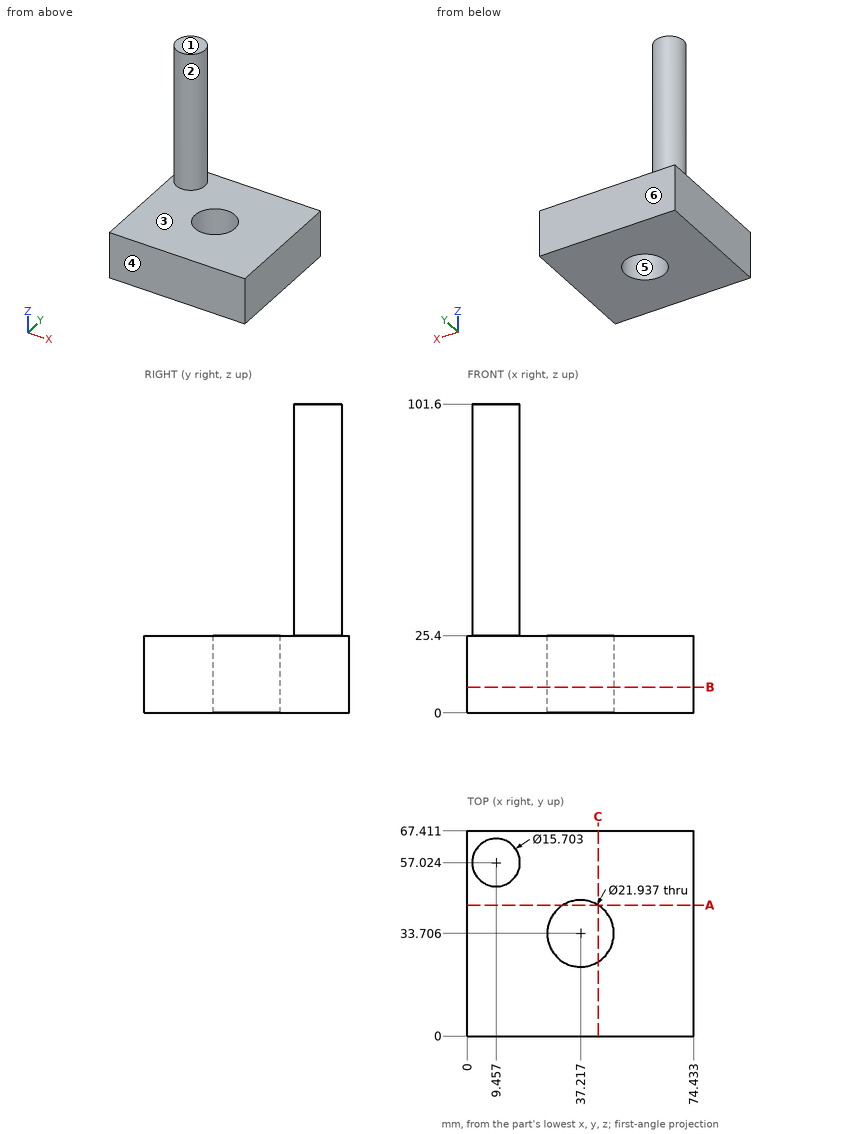
Here's the drawing with two shaded views (mm, measured from the low corner). I have some questions. A direction names the side the tool comes from. Coordinates: 2 decimals unless noted, no trailing zeros. Order: outer loops, then holes, each group sorted by start corner. A loop starts at its lowest first (then second) coordinate and runs counter-clockwise, first axis right, second up.
Item 1: If we mould it in two halves opening along Y, with no side actions, what happens to the marked faces 3, 4, 5 and 6? For each: +Y half, -Y half, draft (parallel to the pull), parting line (faces both ways), or undercut.
Result sheet:
face 3: draft
face 4: -Y half
face 5: undercut
face 6: +Y half
Item 2: If we section it at B-B on z = 8.5: List the corners of the cut face in (x, y) for me (1 decimal).
Result sheet:
outline: (0, 0) - (74.4, 0) - (74.4, 67.4) - (0, 67.4) - close; hole circle Ø21.9 at (37.2, 33.7)
Item 3: If we section it at C-C on x = 43: List the corners of the cut face in (y, z) for me (1 decimal), plus the area to 3 significant figures.
Result sheet:
outline: (0, 0) - (24.4, 0) - (24.4, 25.4) - (0, 25.4) - close; (43, 0) - (67.4, 0) - (67.4, 25.4) - (43, 25.4) - close
area: 1,240 mm2
Item 4: If we section it at A-A on y = 43: List the corners of the cut face in (x, z) for me, plus the area to 3 significant figures.
Result sheet:
outline: (0, 0) - (31.39, 0) - (31.39, 25.4) - (0, 25.4) - close; (43.04, 0) - (74.43, 0) - (74.43, 25.4) - (43.04, 25.4) - close
area: 1,590 mm2
Item 5: For the marked faces 1 and 2, which set-ups out of +Z, -Z, +X, -X, +Y, -Y let a thin tool reach every point of the face, with its end or its side?
Result sheet:
face 1: +Z, +X, -X, +Y, -Y
face 2: +Z
Item 6: I need wall thicknesses on line 1 (Z direction, x = 71, y = 18); line 2 (Y direction, x = 12.5, z = 66) (1 decimal); line 3 (X direction, y = 55.5, z = 67.5) (1 decimal). Which ranges of each line are inside material? Lowest first, please.
Result sheet:
line 1: z = 0 to 25.4
line 2: y = 49.8 to 64.3
line 3: x = 1.8 to 17.2
Item 7: For P1, Ø3, axis at x = 49.5, y = 14, coming from the -Z side, with a flat end and sliding along its axis, tell me the tip position at first contact or that it passes through.
Result sheet:
P1: stops at z = 0
